The figure shows three views and two pictorial views of one solid part (mm, origin at its lowest corner). Answer the questions. A direction names the side the tool comes from. Coordinates: 2 decimals unless noted, no trailing zeros. Write each loop counter-clockwise with the first axis right and the second up, starting at its lowest first coordinate (ties: lowest second). Pieces come first, ordered by that corner, then holes.
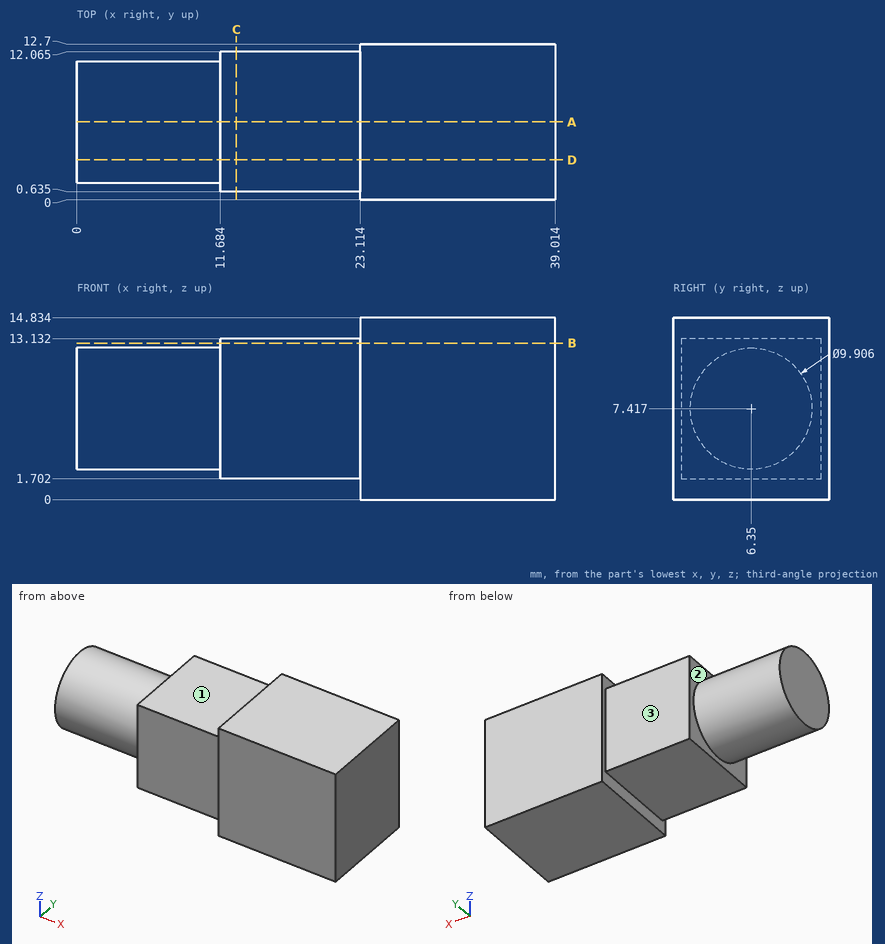
Q1. The part is cut by section C-C, the plane x = 13. Write down the section's boundary in (y, z) (1 decimal), then the cut area to 3 significant figures.
Answers below:
outline: (0.6, 1.7) - (12.1, 1.7) - (12.1, 13.1) - (0.6, 13.1) - close
area: 131 mm2
Q2. Given pin 1 (6 mm diameter, centred on x = 17.5, y = 2.5, fed in from -Z); pin 2 (1.5 mm diameter, centred on y = 3, z = 10.5, fed in from -X), each flat-ended and moving along its own axis, determine where each tip first touches the part or whether it passes through.
Answers below:
pin 1: stops at z = 1.7
pin 2: stops at x = 0
Q3. The part is cut by section D-D, the plane y = 3.25. Write down the section's boundary in (x, z) (1 decimal).
Answers below:
outline: (0, 3.6) - (11.7, 3.6) - (11.7, 1.7) - (23.1, 1.7) - (23.1, 0) - (39, 0) - (39, 14.8) - (23.1, 14.8) - (23.1, 13.1) - (11.7, 13.1) - (11.7, 11.3) - (0, 11.3) - close
Q4. The part is cut by section A-A, the plane y = 6.35. Write down the section's boundary in (x, z) (1 decimal), then the cut area to 3 significant figures.
Answers below:
outline: (0, 2.5) - (11.7, 2.5) - (11.7, 1.7) - (23.1, 1.7) - (23.1, 0) - (39, 0) - (39, 14.8) - (23.1, 14.8) - (23.1, 13.1) - (11.7, 13.1) - (11.7, 12.4) - (0, 12.4) - close
area: 482 mm2
Q5. Which of the six approach directions +Z, -Z, +X, -X, +Y, -Y give full straight-line access (tool end or side, diameter ignored) to the marked faces 1, 2 and 3?
Answers below:
face 1: +Z, -X, +Y, -Y
face 2: -X
face 3: +Z, -Z, -X, +Y
Q6. The part is cut by section B-B, the plane z = 12.75. Write down the section's boundary in (x, y) (1 decimal), then the cut area to 3 significant figures.
Answers below:
outline: (11.7, 0.6) - (23.1, 0.6) - (23.1, 0) - (39, 0) - (39, 12.7) - (23.1, 12.7) - (23.1, 12.1) - (11.7, 12.1) - close
area: 333 mm2
Q7. Find the intervals of material crossed by probe 1 along X at (y, z) = (11.25, 3.5) (1 decimal); probe 2 along Y at (x, z) = (18.5, 10) (1 decimal); probe 3 along Z at (x, y) = (12, 1), in increasing order.
Answers below:
probe 1: x = 11.7 to 39
probe 2: y = 0.6 to 12.1
probe 3: z = 1.7 to 13.13
